```python
from build123d import *

# Parameters (mm, degrees)
F1_DEPTH  = 8
F3_DEPTH  = 5
F4_W      = 3.773983
F4_H      = 38.603006
F4_W_2    = 3.682556
F5_DEPTH  = 5
F6_W      = 75
F6_H      = 3.42278
F7_DEPTH  = 20
F8_W      = 32
F8_H      = 3.133789
F9_DEPTH  = 30
F11_DEPTH = 30
F13_DEPTH = 30
F14_R     = 5
F16_D     = 5


with BuildPart() as f1:
    # F0 (on Top) → F1 (new body)
    with BuildSketch(Plane.XY):
        Polygon((-37.5, -22.5), (37.5, -22.5), (37.5, -11.5), (16, 22.5), (-16, 22.5), (-37.5, -11.5), align=None)
    extrude(amount=F1_DEPTH)

    # F2 (on face) → F3 (cut)
    with BuildSketch(Plane.XY.offset(8)):
        Polygon((-13.546915, 19.525786), (-33.847345, -12.57722), (-33.847345, -19.07722), (34.50483, -19.07722), (34.50483, -12.57722), (14.2044, 19.525786), align=None)
    extrude(amount=-F3_DEPTH, mode=Mode.SUBTRACT)

    # F4 (on face) → F5 (join)
    with BuildSketch(Plane.XY.offset(3)):
        with Locations((-11.659923, 0.224283)):
            Rectangle(F4_W, F4_H)
        with Locations((12.46403, 0.224283)):
            Rectangle(F4_W_2, F4_H)
    extrude(amount=F5_DEPTH)

    # F6 (on face) → F7 (join)
    with BuildSketch(Plane.XY.offset(8)):
        with Locations((0, -20.78861)):
            Rectangle(F6_W, F6_H)
    extrude(amount=F7_DEPTH)

    # F8 (on face) → F9 (join)
    with BuildSketch(Plane.XY.offset(8)):
        with Locations((0, 20.933105)):
            Rectangle(F8_W, F8_H)
    extrude(amount=F9_DEPTH)

    # F10 (on face) → F11 (join)
    with BuildSketch(Plane.XY.offset(8)):
        Polygon((-13.647822, 19.366211), (-16, 22.5), (-30.227941, 0), (-27.132055, -1.957692), align=None)
    extrude(amount=F11_DEPTH)

    # F12 (on face) → F13 (join)
    with BuildSketch(Plane.XY.offset(8)):
        Polygon((16, 22.5), (14.305308, 19.366211), (27.666821, -1.763624), (30.293031, -0.102933), align=None)
    extrude(amount=F13_DEPTH)

    # F14
    f14_edges = [f1.edges().sort_by_distance(p)[0] for p in [
        (0, -22.5, 0),
        (-37.5, -17, 0),
        (37.5, -17, 0),
        (26.75, 5.5, 0),
        (0, 22.5, 0),
        (-26.75, 5.5, 0),
    ]]
    fillet(f14_edges, radius=F14_R)

    # F16 (through all)
    with Locations(Plane(origin=(0, 22.5, 0), x_dir=(-1, 0, 0), z_dir=(0, 1, 0))):
        with Locations((0, 30.490936)):
            Hole(F16_D / 2)


solid = f1.part
```
Design review of the part built by this model. Coordinates are the model's own, in mm. A direction names the side the tool comes from. Give positions to 0.01 mm unless a question says otherwise; leave off trailing zeros. Write each loop counter-clockwise with the first axis right and the second up, starting at its lowest first coordinate (ties: lowest second). Pieces come first, ordered by that corner, then holes.
(1) Add section C-C (x = 1). Give the boundary of the cut face in (y, z), and give its area (3 significant figures).
Checked values:
outline: (-22.5, 5) arc R5 ccw to (-17.5, 0) - (17.5, 0) arc R5 ccw to (22.5, 5) - (22.5, 28.2) - (19.37, 28.2) - (19.37, 8) - (19.53, 8) - (19.53, 3) - (-19.08, 3) - (-19.08, 28) - (-22.5, 28) - close; (19.37, 32.78) - (22.5, 32.78) - (22.5, 38) - (19.37, 38) - close
area: 304 mm2
(2) Add section D-D (x = 9). Give the boundary of the cut face in (y, z).
Checked values:
outline: (-22.5, 5) arc R5 ccw to (-17.5, 0) - (17.5, 0) arc R5 ccw to (22.5, 5) - (22.5, 38) - (19.37, 38) - (19.37, 8) - (19.53, 8) - (19.53, 3) - (-19.08, 3) - (-19.08, 28) - (-22.5, 28) - close
(3) Wall thickness on line 1 along X through (y, z) = (19, 4.5); line 2 along Y through (x, z) = (-10, 15); line 3 along Y through (x, z) = (34, 13): over which ranges is each line inside the solid? List them lowest first.
Checked values:
line 1: x = -18.18 to -13.88, -13.55 to -9.77, 10.62 to 14.31, 14.54 to 18.18
line 2: y = -22.5 to -19.08, 19.37 to 22.5
line 3: y = -22.5 to -19.08
(4) Mouldability with a two-part tool opening along Y and no side actions: class faces 1 (the face through (34.505, -16, 6)), 2 (the face through (0, -4, 0)), 3 (the face through (-0.22, 21.07, 1.5)) as +Y half, -Y half, draft (parallel to the pull), parting line (faces both ways), or undercut.
Checked values:
face 1: undercut
face 2: draft
face 3: +Y half
(5) Add section B-B (z = 6.5). Give the boundary of the cut face in (x, y).
Checked values:
outline: (-37.5, -22.5) - (37.5, -22.5) - (37.5, -11.5) - (16, 22.5) - (-16, 22.5) - (-37.5, -11.5) - close; hole (-33.85, -19.08) - (-13.55, -19.08) - (-13.55, 19.53) - (-33.85, -12.58) - close; hole (-9.77, -19.08) - (10.62, -19.08) - (10.62, 19.53) - (-9.77, 19.53) - close; hole (14.31, -19.08) - (34.5, -19.08) - (34.5, -12.58) - (14.31, 19.37) - close
(6) Clearance check with flat-ended pins moving along their axes: pin 1 Ø6 at (x, y) = (3.5, 8) entering from +Z; pin 2 Ø3 at (x, y) = (-12, 8) entering from +Z; pin 3 Ø12 at (y, z) = (-7, 28) entering from -X. State where each tip first meets the part, or that it passes through.
Checked values:
pin 1: stops at z = 3
pin 2: stops at z = 8
pin 3: stops at x = -28.65
(7) Tool access review of faces 4 (the face through (28.962, -0.945, 22.79)), 5 (the face through (1, 19.526, 6)), 6 (the face through (-1, -22.5, 16)), 7 (the face through (-2, 20, 38)), 8 (the face through (-1, -19.077, 15)): name each direction out of +Z, -Z, +X, -X, +Y, -Y from which nothing blocks a thin tool from reaching the whole face with its end or side.
Checked values:
face 4: +Z, +X
face 5: none
face 6: +Z, -Z, +X, -X, -Y
face 7: +Z, +X, -X, +Y, -Y
face 8: +Z
(8) Add section A-A (z = 10.5). Give the boundary of the cut face in (x, y).
Checked values:
outline: (-37.5, -22.5) - (37.5, -22.5) - (37.5, -19.08) - (-37.5, -19.08) - close; (-30.23, 0) - (-27.13, -1.96) - (-13.65, 19.37) - (14.31, 19.37) - (27.67, -1.76) - (30.29, -0.1) - (16, 22.5) - (-16, 22.5) - close
